Verification items for this drawing (mm, ordinates from the low corner). A direction names the side the tool comes from. Round coordinates to 2 decimals unless told otherwise and drop trailing zeros. Order: outer loops, then holes, each group sorted by start corner. A loop starts at its lowest first (then second) coordinate and runs counter-clockwise, first axis right, second up. Notation, with made-up numbers: (-24, -21.5) -> (31, -21.5) arc R31 ccw to (31, 6.5) -> close; hole circle Ø7 at (-18, 59.5). An arc over 180 degrees is marked (long way). Use a Markdown table: item, result. Add a question column.
Item 1: Sectioned sample at C-C, the plane y = 12.25. Record the cut outline in (x, z).
Item 2: Material ranges on probe 1 along Y at (x, z) = (13, 0.2); probe 2 along X at (y, z) = (12.5, 1), recorded low to high. Write a range as [from, to].
Item 3: Sectioned sample at B-B, the plane z = 1.25. Record the cut outline in (x, y), and give its area (3 significant figures).
Item 4: Gauge pin test, flat ends, axial feed: pin 1 Ø0.9 at (x, z) = (2, 2) entering from +Y; pin 2 Ø1.5 at (y, z) = (5.5, 1.5) entering from -X; pin 3 Ø1.5 at (y, z) = (12.5, 2) entering from +X. Record the tip position at first contact, or that the pin passes through.
Item 5: Sectioned sample at A-A, the plane x = 12. Record the cut outline in (y, z), and give its area (3 significant figures).
Item 6: Set-up check for the marked faces 1, 2 and 3: record each of +Z, -Z, +X, -X, +Y, -Y from which the full face is reachable in a straight line by a thin tool's end or side.
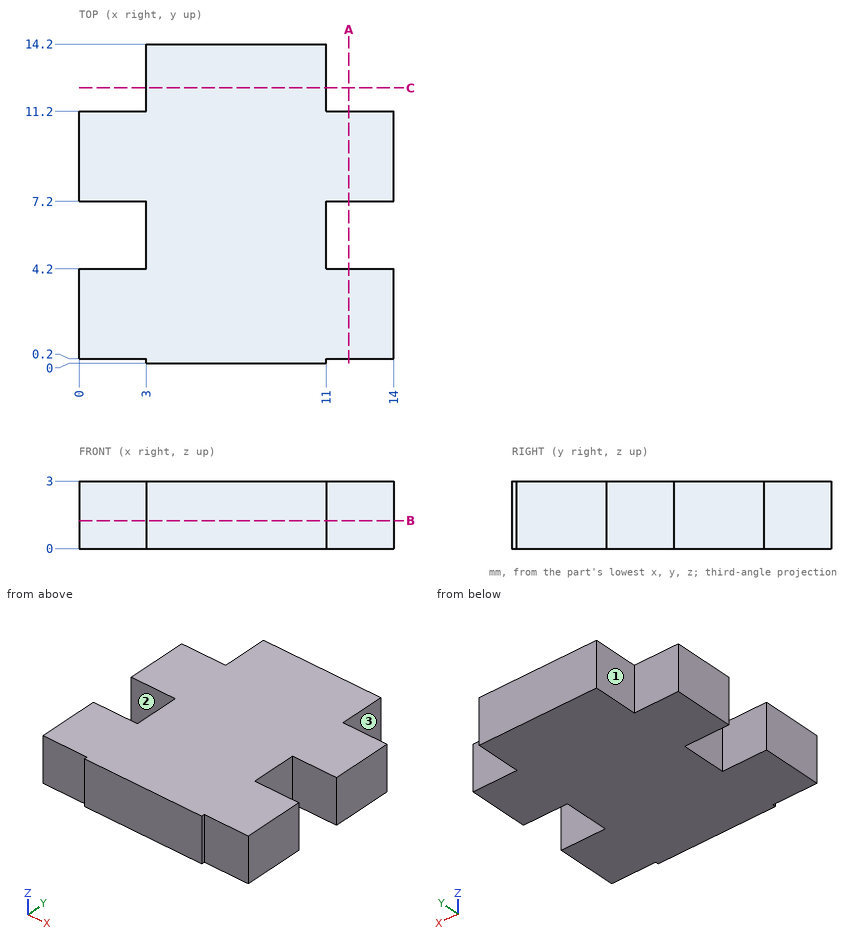
Found:
| question | item | result |
|---|---|---|
| 1 | outline | (3, 0) -> (11, 0) -> (11, 3) -> (3, 3) -> close |
| 2 | probe 1 | y = [0.2, 4.2], [7.2, 11.2] |
| 2 | probe 2 | x = [3, 11] |
| 3 | outline | (0, 0.2) -> (3, 0.2) -> (3, 0) -> (11, 0) -> (11, 0.2) -> (14, 0.2) -> (14, 4.2) -> (11, 4.2) -> (11, 7.2) -> (14, 7.2) -> (14, 11.2) -> (11, 11.2) -> (11, 14.2) -> (3, 14.2) -> (3, 11.2) -> (0, 11.2) -> (0, 7.2) -> (3, 7.2) -> (3, 4.2) -> (0, 4.2) -> close |
| 3 | area | 162 mm2 |
| 4 | pin 1 | stops at y = 11.2 |
| 4 | pin 2 | stops at x = 3 |
| 4 | pin 3 | stops at x = 11 |
| 5 | outline | (0.2, 0) -> (4.2, 0) -> (4.2, 3) -> (0.2, 3) -> close; (7.2, 0) -> (11.2, 0) -> (11.2, 3) -> (7.2, 3) -> close |
| 5 | area | 24.0 mm2 |
| 6 | face 1 | +Z, -Z, -X, +Y |
| 6 | face 2 | +Z, -Z, -X |
| 6 | face 3 | +Z, -Z, +X, +Y |
